from build123d import *

# Parameters (mm, degrees)
FILLET1_R          = 4.064
SKETCH10_W         = 2.857500069
SKETCH10_H         = 7.5184
REVOLVE3_ANGLE     = 20
CUT_EXTRUDE1_START = 1.27
CUT_EXTRUDE1_DEPTH = 4.9784
CIRPATTERN4_COUNT  = 2
FILLET8_R          = 1.27
FILLET9_R          = 1.27


with BuildPart() as part:
    # Sketch1 → Revolve1 (revolve)
    with BuildSketch(Plane.XY, mode=Mode.PRIVATE) as revolve1_sk:
        Polygon((0, 9.1059), (-20.6375, 9.1059), (-20.6375, 5.042647059), (-17.78, 5.042647059), (-17.78, -5.042647059), (-20.6375, -5.042647059), (-20.6375, -19.7231), (-16.51, -19.7231), (-16.51, -15.5956), (-18.0975, -15.5956), (-18.0975, -13.3096), (-16.51, -13.3096), (-16.51, 6.7564), (-3.8481, 6.7564), (-3.0861, 7.5184), (0, 7.5184), align=None)
    revolve(revolve1_sk.sketch.rotate(Axis((0, 0, 0), (0, 1, 0)), 270), axis=Axis((0, 0, 0), (0, 1, 0)))

    # Fillet1
    # the kernel refuses this fillet: 4.064 mm, written as the material it takes off along each edge
    with BuildSketch(Plane(origin=(0, 9.1059, 0), x_dir=(0, 0, -1), z_dir=(1, 0, 0))) as fillet1_piece_1:
        with BuildLine():
            CenterArc((16.573500069, -4.064), FILLET1_R, 0.010532312, 89.989467688)
            Line((20.6375, -4.063252941), (20.718779999, -4.063238))
            Line((20.718779999, -4.063238), (20.71878, 0))
            Line((20.71878, 0), (20.6375, 0.08128))
            Line((20.6375, 0.08128), (16.573500069, 0.08128))
            Line((16.573500069, 0.08128), (16.573500069, 0))
        make_face()
    revolve(axis=Axis((0, 9.1059, 0), (0, 1, 0)), mode=Mode.SUBTRACT)

    # Sketch10 → Revolve3 (revolve, symmetric)
    with BuildSketch(Plane.XY) as revolve3_sk:
        with Locations((-19.208750034, 0)):
            Rectangle(SKETCH10_W, SKETCH10_H)
    revolve3 = revolve(axis=Axis((0, 0, 0), (0, 1, 0)), revolution_arc=REVOLVE3_ANGLE / 2)
    revolve3 = revolve3 + revolve(revolve3_sk.sketch, axis=Axis((0, 0, 0), (0, -1, 0)), revolution_arc=REVOLVE3_ANGLE / 2)

    # Sketch12 → Cut-Extrude1 (cut)
    with BuildSketch(Plane(origin=(0, -3.7592, 0), x_dir=(1, 0, 0), z_dir=(0, 1, 0)).offset(CUT_EXTRUDE1_START)):
        with BuildLine():
            Line((-7.313638514, 0), (-17.215440903, 1.745954919))
            ThreePointArc((-17.215440903, 1.745954919), (-17.30375, 0), (-17.215440903, -1.745954919))
            Line((-17.215440903, -1.745954919), (-7.313638514, 0))
        make_face()
    cut_extrude1 = extrude(amount=CUT_EXTRUDE1_DEPTH, mode=Mode.SUBTRACT)

    # CirPattern4: Revolve3, Cut-Extrude1 ×2 about axis
    cirpattern4_axis = Axis((0, 0, 0), (0, 1, 0))
    add([revolve3.rotate(cirpattern4_axis, i * 360 / CIRPATTERN4_COUNT) for i in range(1, CIRPATTERN4_COUNT)])
    add([cut_extrude1.rotate(cirpattern4_axis, i * 360 / CIRPATTERN4_COUNT) for i in range(1, CIRPATTERN4_COUNT)], mode=Mode.SUBTRACT)

    # Fillet8
    # the kernel refuses this fillet: 1.27 mm, written as the material it takes off along each edge
    with BuildSketch(Plane(origin=(-16.431533746, -2.4892, -1.607730937), x_dir=(0.1324793231915166, 0, -0.9911857691304479), z_dir=(0, 1, 0)), Plane(origin=(16.431533746, -2.4892, 1.607730937), x_dir=(-0.13247932319151873, 0, 0.9911857691304475), z_dir=(0, 1, 0))) as fillet8_piece_1:
        with BuildLine():
            CenterArc((1.211424462, 1.269207194), FILLET8_R, 201.909884157, 66.065503548)
            Line((0.033154154, 0.795309438), (0.009588748, 0.785831483))
            ThreePointArc((0.009588748, 0.785831483), (-0.008800881, 0.398712653), (-0.025377958, 0.001057934))
            Line((-0.025377958, 0.001057934), (0.000897351, -0.025384144))
            ThreePointArc((0.000897351, -0.025384144), (0.583278445, -0.01509352), (1.165659538, -0.025384144))
            Line((1.165659538, -0.025384144), (1.166556889, 0))
        make_face()
    extrude(amount=4.9784, mode=Mode.SUBTRACT)
    with BuildSketch(Plane(origin=(-16.431533746, -2.4892, 1.607730937), x_dir=(0.13247932319152245, 0, 0.9911857691304472), z_dir=(0, 1, 0)), Plane(origin=(16.431533746, -2.4892, -1.607730937), x_dir=(-0.13247932319151992, 0, -0.9911857691304475), z_dir=(0, 1, 0))) as fillet8_piece_2:
        with BuildLine():
            CenterArc((1.211424462, -1.269207194), FILLET8_R, 92.024612295, 66.065503548)
            Line((0.033154154, -0.795309438), (0.009588748, -0.785831483))
            ThreePointArc((0.009588748, -0.785831483), (-0.008800881, -0.398712653), (-0.025377958, -0.001057934))
            Line((-0.025377958, -0.001057934), (0.000897351, 0.025384144))
            ThreePointArc((0.000897351, 0.025384144), (0.583278445, 0.01509352), (1.165659538, 0.025384144))
            Line((1.165659538, 0.025384144), (1.166556889, 0))
        make_face()
    extrude(amount=4.9784, mode=Mode.SUBTRACT)

    # Fillet9
    fillet9_edges = [part.edges().sort_by_distance(p)[0] for p in [
        (-17.215440903, 0, 1.745954919),
        (-17.215440903, 0, -1.745954919),
        (17.215440903, 0, -1.745954919),
        (17.215440903, 0, 1.745954919),
    ]]
    fillet(fillet9_edges, radius=FILLET9_R)


solid = part.part
Verification items for the finished model (mm, model axes). A direction names the side the tool comes from. Coordinates: 2 decimals unless noted, no trailing zeros. Order: outer loops, then holes, each group sorted by start corner. A loop starts at its lowest first (then second) coordinate and runs counter-clockwise, first axis right, second up. Notation, with made-up numbers: M 89,25 L 114,25 A29 cw 114,60 Z; hole C 17.25,79 d3. An arc over 180 degrees is marked long. Return JSON: item names as keys, results as strings.
1) Cross-section at A-A, the plane x = 0. Record the boundary of the cut face in (y, z), and give its area (3 significant figures).
Answer list:
{"outline": "M -19.72,-20.64 L -5.04,-20.64 L -5.04,-17.78 L 5.04,-17.78 L 5.04,-20.64 A4.06 ccw 9.11,-16.57 L 9.11,16.57 A4.06 ccw 5.04,20.64 L 5.04,17.78 L -5.04,17.78 L -5.04,20.64 L -19.72,20.64 L -19.72,16.51 L -15.6,16.51 L -15.6,18.1 L -13.31,18.1 L -13.31,16.51 L 6.76,16.51 L 6.76,3.85 L 7.52,3.09 L 7.52,-3.09 L 6.76,-3.85 L 6.76,-16.51 L -13.31,-16.51 L -13.31,-18.1 L -15.6,-18.1 L -15.6,-16.51 L -19.72,-16.51 Z", "area": "238 mm2"}
2) Cross-section at B-B, the plane y = -12.75. Record the boundary of the cut face in (x, z) (1 decimal).
Answer list:
{"outline": "C 0,0 d41.3; hole C 0,0 d33"}
3) Thickness scan on L1, parallel to X at y = -15, z = 0; L2, parallel to X at y = -6.25, z = 0; L3, parallel to Y at x = -6, z = -5.5. Record the ranges inside material, lowest first. Write a range as [from, to].
Answer list:
{"L1": "[-20.64, -18.1], [18.1, 20.64]", "L2": "[-20.64, -16.51], [16.51, 20.64]", "L3": "[6.76, 9.11]"}
4) Gauge pin test, flat ends, axial feed: pin 1 (2 mm diameter, centred on x = -9.5, y = -13, fed in from -Z); pin 2 (1 mm diameter, centred on y = -6.5, z = 8.5, fed in from -X); pin 3 (2.5 mm diameter, centred on x = 19, z = 0, fed in from +Y). Record the tip position at first contact, or that the pin passes through.
Answer list:
{"pin 1": "z = -18.81", "pin 2": "x = -19.02", "pin 3": "y = 8.93"}
5) Release check for a two-part mould opening along Y. For faces 1 (the flat face through (-18.94, 0.05, -3.34)), 2 (the cylindrical face through (10.05, -17.63, 13.1)), 3 (the flat face through (0, 9.106, 0)), 4 (the cylindrical face through (17.36, -0.07, 3.85)) record: +Y half, -Y half, draft (parallel to the pull), parting line (faces both ways), or undercut.
Answer list:
{"face 1": "undercut", "face 2": "draft", "face 3": "+Y half", "face 4": "undercut"}
6) Access from +Z, -Z, +X, -X, +Y, -Y to the whole of each face (thin tool, end or side, straight path). Record for faces 5 (the flat face through (0, 6.756, 4)), 6 (the flat face through (-18.94, 0.05, 3.34)), 7 (the flat face through (-13.9, -19.723, 9.3)), 8 (the cylindrical face through (17.304, -0.035, 0.014)).
Answer list:
{"face 5": "-Y", "face 6": "+Z", "face 7": "+Z, -Z, +X, -X, -Y", "face 8": "none"}
